Check sheet for the modelled part. Datum: model origin and axes. Units: mm. A direction names the side the tool comes from. Coordinates: 2 decimals unless noted, no trailing zeros. Loops run counter-clockwise (first coordinate to the right, second up) from the corner with the lowest first, then second, coordinate; pieces in that order, holes last. Notation, with made-up numbers: (-15, 52) -> (10, 52) arc R7 cw to (10, 59) -> close; hole circle Ø9 at (33, 83.5). An arc over 180 degrees is marked (long way). Use CSV: the item, a comma, the result in double quotes. Start each with the question number.
1. Release check for a two-part mould opening along X. For faces 1 (the face through (58.5, 17, 3)), 2 (the face through (60, 17, 3)), 3 (the face through (32, 34, 3.7)) record: pulls with the +X half, pulls with the -X half, needs draft (parallel to the pull), parting line crosses it, or undercut.
2. Sectioned sample at A-A, the plane y = 25. Record the cut outline in (x, z).
3. Gauge pin test, flat ends, axial feed: pin 1 (3 mm diameter, centred on x = 36, y = 22.5, fed in from +Z); pin 2 (1.3 mm diameter, centred on y = 17.5, z = 3, fed in from +X); pin 3 (0.6 mm diameter, centred on x = 36, z = 3, fed in from +Y). Record the tip position at first contact, or that the pin passes through.
4. Sectioned sample at B-B, the plane x = 51. Record the cut outline in (y, z), and give its area (3 significant figures).
5. Thickness scan on L1, parallel to X at y = 24.5, z = 3.25; L2, parallel to Z at x = 52.5, y = 25; L3, parallel to X at y = 1, z = 2.95. Record the ranges inside material, lowest first.
6. Set-up check for faces 4 (the face through (30, 1.5, 3)), 5 (the face through (30, 0, 3)), 6 (the face through (30, 35, 3)), 7 (the face through (30, 18, 0)), 8 (the face through (0, 18, 3)): record each of +Z, -Z, +X, -X, +Y, -Y from which the full face is reachable in a straight line by a thin tool's end or side.
Autodesk Fusion 360 part; units mm, degrees
sketch "Skizze2" plane through (0, 0, 0) normal (0, 0, 1) x (1, 0, 0)
  line L0 (-2.5, 35) -> (-2.5, 37.5)
  line L1 (-2.5, 37.5) -> (0, 37.5)
  line L2 (62.5, 0) -> (62.5, -2.5)
  line L3 (62.5, -2.5) -> (60, -2.5)
  line L4 (-2.5, 37.5) -> (62.5, 37.5)
  line L5 (62.5, 37.5) -> (62.5, -2.5)
  line L6 (62.5, -2.5) -> (-2.5, -2.5)
  line L7 (-2.5, -2.5) -> (-2.5, 37.5)
  point P0 (0, 35)
  point P1 (60, 0)
  dimension "d3" = 2.5
  dimension "d4" = 2.5
  dimension "d5" = 2.5
  dimension "d6" = 2.5
extrude "Extrusion1" add sketch "Skizze2" along normal blind 2.5
sketch "Skizze3" plane through (0, 0, 2.5) normal (0, 0, 1) x (-1, 0, 0)
  line L0 (2.5, 2.5) -> (-62.5, 2.5)
  line L1 (-62.5, 2.5) -> (-62.5, -37.5)
  line L2 (-62.5, -37.5) -> (2.5, -37.5)
  line L3 (2.5, -37.5) -> (2.5, 2.5)
  line L4 (-62.5, -37.5) -> (-60, -37.5)
  line L5 (-62.5, -35) -> (-62.5, -37.5)
  line L6 (2.5, 2.5) -> (0, 2.5)
  line L7 (2.5, 0) -> (2.5, 2.5)
  line L8 (0, 0) -> (-60, 0)
  line L9 (-60, 0) -> (-60, -35)
  line L10 (-60, -35) -> (0, -35)
  line L11 (0, -35) -> (0, 0)
  dimension "d9" = 2.5
  dimension "d10" = 2.5
  dimension "d11" = 2.5
  dimension "d12" = 2.5
extrude "Extrusion2" add sketch "Skizze3" along normal blind 2 contours L8 L9 L10 L11
sketch "Skizze4" plane through (0, 0, 4.5) normal (0, 0, 1) x (-1, 0, 0)
  line L0 (0, -35) -> (0, 0)
  line L1 (0, 0) -> (-60, 0)
  line L2 (-60, 0) -> (-60, -35)
  line L3 (-60, -35) -> (0, -35)
  line L4 (-1.5, -1.5) -> (-58.5, -1.5)
  line L5 (-58.5, -1.5) -> (-58.5, -33.5)
  line L6 (-58.5, -33.5) -> (-1.5, -33.5)
  line L7 (-1.5, -33.5) -> (-1.5, -1.5)
extrude "Extrusion3" cut sketch "Skizze4" against normal blind 2 contours L4 L5 L6 L7
extrude "Extrusion4" cut 1 faces at (39.5, 0.5, 4.5) along direction (0, 0, -1) blind 0.8
Completed:
1,face 1,"undercut"
1,face 2,"pulls with the +X half"
1,face 3,"needs draft"
2,outline,"(-2.5, 0) -> (62.5, 0) -> (62.5, 2.5) -> (60, 2.5) -> (60, 3.7) -> (58.5, 3.7) -> (58.5, 2.5) -> (1.5, 2.5) -> (1.5, 3.7) -> (0, 3.7) -> (0, 2.5) -> (-2.5, 2.5) -> close"
3,pin 1,"z = 2.5"
3,pin 2,"x = 62.5"
3,pin 3,"y = 35"
4,outline,"(-2.5, 0) -> (37.5, 0) -> (37.5, 2.5) -> (35, 2.5) -> (35, 3.7) -> (33.5, 3.7) -> (33.5, 2.5) -> (1.5, 2.5) -> (1.5, 3.7) -> (0, 3.7) -> (0, 2.5) -> (-2.5, 2.5) -> close"
4,area,"104 mm²"
5,L1,"0 to 1.5, 58.5 to 60"
5,L2,"0 to 2.5"
5,L3,"0 to 60"
6,face 4,"+Z"
6,face 5,"+Z, +X, -X, -Y"
6,face 6,"+Z, +X, -X, +Y"
6,face 7,"-Z, +X, -X, +Y, -Y"
6,face 8,"+Z, -X, +Y, -Y"
